Verification items for the finished model (mm, model axes). A direction names the side the tool comes from. Round coordinates to 2 decimals unless told otherwise and drop trailing zeros. Loops run counter-clockwise (first coordinate to the right, second up) from the corner with the lowest first, then second, coordinate; pieces in that order, holes last. Notation, with made-up numbers: (78.5, 74.25) -> (122.5, 74.25) arc R34 cw to (122.5, 104.25) -> close; hole circle Ø1 at (-39.5, 17.5). An arc over 180 degrees is marked (long way). Use a Markdown table: item, result. Add a question column.
```python
from build123d import *

# Parameters (mm, degrees)
BOSS_EXTRUDE1_DEPTH = 32
FILLET1_R           = 10
FILLET2_R           = 10
BOSS_EXTRUDE2_DEPTH = 19
SKETCH3_R           = 12
CUT_EXTRUDE1_DEPTH  = 19
SKETCH4_R           = 20
CUT_EXTRUDE2_DEPTH  = 9.5
SKETCH5_W           = 146.165275263
SKETCH5_H           = 22
CUT_EXTRUDE3_DEPTH  = 6
SKETCH6_W           = 22
SKETCH6_H           = 63.302471394
CUT_EXTRUDE4_DEPTH  = 6
SKETCH7_W           = 70
SKETCH7_H           = 21.06948543
BOSS_EXTRUDE3_DEPTH = 25
BOSS_EXTRUDE4_DEPTH = 70
SKETCH9_R           = 5
CUT_EXTRUDE5_DEPTH  = 70
SKETCH10_W          = 40
SKETCH10_H          = 90
CUT_EXTRUDE6_DEPTH  = 70


with BuildPart() as part:
    # Sketch1 → Boss-Extrude1 (new, symmetric)
    with BuildSketch(Plane.XY):
        Polygon((0, 0), (140, 0), (140, 19), (25.626336332, 19), (-4.402994998, 48.830779291), (34.987574414, 70.857602718), (23.194010005, 86.289579595), (-32, 55.425625842), align=None)
    extrude(amount=BOSS_EXTRUDE1_DEPTH, both=True)

    # Fillet1
    fillet1_edges = [part.edges().sort_by_distance(p)[0] for p in [
        (-4.402994998, 48.830779291, 0),
    ]]
    fillet(fillet1_edges, radius=FILLET1_R)

    # Fillet2
    fillet2_edges = [part.edges().sort_by_distance(p)[0] for p in [
        (25.626336332, 19, 0),
    ]]
    fillet(fillet2_edges, radius=FILLET2_R)

    # Sketch2 → Boss-Extrude2 (add)
    with BuildSketch(Plane(origin=(-31.233234019, 55.854393924, 0), x_dir=(0.8728071364976854, 0.4880652645689006, 0), z_dir=(-0.48806526456890054, 0.8728071364976853, 0))):
        with BuildLine():
            ThreePointArc((62.358843951, 32), (94.358843951, 0), (62.358843951, -32))
            Line((62.358843951, -32), (62.358843951, 32))
        make_face()
    extrude(amount=-BOSS_EXTRUDE2_DEPTH)

    # Sketch3 → Cut-Extrude1 (cut)
    with BuildSketch(Plane(origin=(-31.233234019, 55.854393924, 0), x_dir=(0.8728071364976854, 0.4880652645689006, 0), z_dir=(-0.48806526456890054, 0.8728071364976853, 0))):
        with Locations(Location((62.358843951, 0, 0), (0, 0, 180))):
            Circle(SKETCH3_R)
    extrude(amount=-CUT_EXTRUDE1_DEPTH, mode=Mode.SUBTRACT)

    # Sketch4 → Cut-Extrude2 (cut)
    with BuildSketch(Plane(origin=(-31.233234019, 55.854393924, 0), x_dir=(0.8728071364976854, 0.4880652645689006, 0), z_dir=(-0.48806526456890054, 0.8728071364976853, 0))):
        with Locations(Location((62.358843951, 0, 0), (0, 0, 180))):
            Circle(SKETCH4_R)
    extrude(amount=-CUT_EXTRUDE2_DEPTH, mode=Mode.SUBTRACT)

    # Sketch5 → Cut-Extrude3 (cut)
    with BuildSketch(Plane(origin=(-31.233234019, 55.854393924, 0), x_dir=(0.8728071364976854, 0.4880652645689006, 0), z_dir=(-0.48806526456890054, 0.8728071364976853, 0))):
        with Locations((62.35884395, 0)):
            Rectangle(SKETCH5_W, SKETCH5_H)
    extrude(amount=-CUT_EXTRUDE3_DEPTH, mode=Mode.SUBTRACT)

    # Sketch6 → Cut-Extrude4 (cut)
    with BuildSketch(Plane(origin=(0, 0, 0), x_dir=(0, 0, 1), z_dir=(-0.8660254037844362, -0.5000000000000046, 0))):
        with Locations((0, 57.999434657)):
            Rectangle(SKETCH6_W, SKETCH6_H)
    extrude(amount=-CUT_EXTRUDE4_DEPTH, mode=Mode.SUBTRACT)

    # Sketch7 → Boss-Extrude3 (add)
    with BuildSketch(Plane(origin=(0, 19, 0), x_dir=(1, 0, 0), z_dir=(0, 1, 0))):
        with Locations((85.152528748, 0)):
            Rectangle(SKETCH7_W, SKETCH7_H)
    extrude(amount=BOSS_EXTRUDE3_DEPTH)

    # Sketch8 → Boss-Extrude4 (add)
    with BuildSketch(Plane(origin=(120.152528748, 0, 0), x_dir=(0, 0, -1), z_dir=(1, 0, 0))):
        with BuildLine():
            ThreePointArc((-10.534742715, 44), (0, 54.534742715), (10.534742715, 44))
            Line((10.534742715, 44), (-10.534742715, 44))
        make_face()
    extrude(amount=-BOSS_EXTRUDE4_DEPTH)

    # Sketch9 → Cut-Extrude5 (cut)
    with BuildSketch(Plane(origin=(120.152528748, 0, 0), x_dir=(0, 0, -1), z_dir=(1, 0, 0))):
        with Locations(Location((0, 44, 0), (0, 0, 90))):
            Circle(SKETCH9_R)
    extrude(amount=-CUT_EXTRUDE5_DEPTH, mode=Mode.SUBTRACT)

    # Sketch10 → Cut-Extrude6 (cut)
    with BuildSketch(Plane.XY.offset(10.534742715)):
        with Locations((85.152528748, 70.106665045)):
            Rectangle(SKETCH10_W, SKETCH10_H)
    extrude(amount=-CUT_EXTRUDE6_DEPTH, mode=Mode.SUBTRACT)


solid = part.part
```
1) Go/stop test with flat-tipped pins: pin 1 (1 mm diameter, centred on x = 103, z = 11, fed in from +Y); pin 2 (1.5 mm diameter, centred on x = 49.5, z = -19, fed in from -Y); pin 3 (10.5 mm diameter, centred on y = 43.5, z = -3, fed in from -X); pin 4 (23 mm diameter, centred on y = 40.5, z = -0.5, fed in from +X). Record where each tip stops, or that it passes through.
2) Thickness scan on line 1 (Z direction, x = 54.25, y = 44); line 2 (X direction, y = 52.5, z = 4); line 3 (Y direction, x = 95.5, z = -23.5). Record the ranges inside material, lowest first.
3) Sectioned sample at D-D on y = 58.5. Enter the section's corners in (x, z), then the cut area to 3 significant figures.
4) Access from +Z, -Z, +X, -X, +Y, -Y to the whole of each face (thin tool, end or side, straight path). Record for faces 4 (the face through (20.886, 62.972, 0.448)), 5 (the face through (105.153, 36, 0)), 6 (the face through (45, 95, 11)), 7 (the face through (-18, 57, -11)), 8 (the face through (120.153, 33, 0)).
5) Sectioned sample at C-C on x = 88.5. Enter the section's corners in (y, z).
6) Sectioned sample at A-A on x = 107. Enter the section's corners in (y, z), then the cut area to 3 significant figures.
7) Release check for a two-part mould opening along Z. For faces 1 (the face through (-15.98, 39.68, -0.15)), 2 (the face through (57.758, 54.532, 0.232)), 3 (the face through (85, 23, 10.535)) record: released by +Z, released by -Z, zero draft, split by the parting line, or undercut.
Geometry results:
| question | item | result |
|---|---|---|
| 1 | pin 1 | y = 25.11 |
| 1 | pin 2 | y = 0 |
| 1 | pin 3 | x = -21.22 |
| 1 | pin 4 | x = 120.15 |
| 2 | line 1 | -10.53 to -5, 5 to 10.53 |
| 2 | line 2 | -23.38 to 4, 50.15 to 65.15, 105.15 to 120.15 |
| 2 | line 3 | 0 to 19 |
| 3 | outline | (-26.5, -32) -> (12.89, -32) -> (12.89, 32) -> (-26.5, 32) -> (-26.5, 11) -> (-14.21, 11) -> (-14.21, -11) -> (-26.5, -11) -> close |
| 3 | area | 2,250 mm^2 |
| 4 | face 4 | +Z, -Z, +X |
| 4 | face 5 | +Z, -Z, +Y |
| 4 | face 6 | -X, +Y |
| 4 | face 7 | -X |
| 4 | face 8 | +Z, -Z, +X, +Y |
| 5 | outline | (0, -32) -> (19, -32) -> (19, -10.53) -> (25.11, -10.53) -> (25.11, 10.53) -> (19, 10.53) -> (19, 32) -> (0, 32) -> close |
| 6 | outline | (0, -32) -> (19, -32) -> (19, -10.53) -> (44, -10.53) arc R10.53 ccw to (44, 10.53) -> (19, 10.53) -> (19, 32) -> (0, 32) -> close; hole circle Ø10 at (44, 0) |
| 6 | area | 1,840 mm^2 |
| 7 | face 1 | undercut |
| 7 | face 2 | split by the parting line |
| 7 | face 3 | released by +Z |
